Part model, mm, in its own coordinate system. Give positions to 0.01 mm unless a question says otherwise; leave off trailing zeros. Write each loop counter-clockwise with the first axis right and the second up, starting at its lowest first coordinate (ties: lowest second). Pieces come first, ordered by that corner, then holes. Notation, with made-up numbers: M 53.25,7.25 L 73.25,7.25 A7 ccw 73.25,14.25 Z; hole C 50,73.25 d8. An arc over 180 degrees is marked long. Use a Markdown table: item, result.
```python
from build123d import *

# Parameters (mm, degrees)
SKETCH1_W               = 22.86
SKETCH1_H               = 20.32
BOSS_EXTRUDE1_DEPTH     = 0.635
SKETCH2_R               = 1
CUT_EXTRUDE1_DEPTH      = 1
CUT_EXTRUDE1_DEPTH_BACK = 2.27


with BuildPart() as part:
    # Sketch1 → Boss-Extrude1 (new body, symmetric)
    with BuildSketch(Plane(origin=(0, 0, 0), x_dir=(1, 0, 0), z_dir=(0, 1, 0))):
        Rectangle(SKETCH1_W, SKETCH1_H)
    extrude(amount=BOSS_EXTRUDE1_DEPTH, both=True)

    # Sketch2 → Cut-Extrude1 (cut, two sides)
    with BuildSketch(Plane(origin=(0, 0.635, 0), x_dir=(1, 0, 0), z_dir=(0, 1, 0))) as cut_extrude1_sk:
        with Locations((-8.89, 7.62)):
            Circle(SKETCH2_R)
        with Locations((8.89, 7.62)):
            Circle(SKETCH2_R)
    extrude(amount=CUT_EXTRUDE1_DEPTH, mode=Mode.SUBTRACT)
    extrude(cut_extrude1_sk.sketch, amount=-CUT_EXTRUDE1_DEPTH_BACK, mode=Mode.SUBTRACT)


solid = part.part
```
1. Two-plate mould, pull along Z, no slides. Class faces 1 (the cylindrical face through (8.153, 0.009, -8.296)), 2 (the flat face through (0, 0, -10.16)), 3 (the flat face through (-11.43, 0, 0)): released by +Z, released by -Z, zero draft, split by the parting line, or undercut.
Findings below:
| item | result |
|---|---|
| face 1 | undercut |
| face 2 | released by -Z |
| face 3 | zero draft |
2. Cut at B-B, the plane z = -7.62. Give the cut face in (x, y) (3 decimals).
Findings below:
| item | result |
|---|---|
| outline | M -11.43,-0.635 L -9.89,-0.635 L -9.89,0.635 L -11.43,0.635 Z; M -7.89,-0.635 L 7.89,-0.635 L 7.89,0.635 L -7.89,0.635 Z; M 9.89,-0.635 L 11.43,-0.635 L 11.43,0.635 L 9.89,0.635 Z |
3. Drill centre lines: L1, parallel to X at y = 0.15, z = -7.62; L2, parallel to X at y = -0.05, z = -6.75; L3, parallel to Z at x = -8.89, y = -0.1. Where is each one in solid material? Low to high.
Findings below:
| item | result |
|---|---|
| L1 | -11.43 to -9.89, -7.89 to 7.89, 9.89 to 11.43 |
| L2 | -11.43 to -9.38, -8.4 to 8.4, 9.38 to 11.43 |
| L3 | -10.16 to -8.62, -6.62 to 10.16 |
4. Cut at A-A, the plane x = 8.89. Give the cut face in (y, z) (3 decimals).
Findings below:
| item | result |
|---|---|
| outline | M -0.635,-10.16 L 0.635,-10.16 L 0.635,-8.62 L -0.635,-8.62 Z; M -0.635,-6.62 L 0.635,-6.62 L 0.635,10.16 L -0.635,10.16 Z |
